Autodesk Inventor part; units mm, degrees
ref_plane "YZ Plane" through (0, 0, 0) normal (1, 0, 0) x (0, 1, 0)
ref_plane "XZ Plane" through (0, 0, 0) normal (0, 1, 0) x (-1, 0, 0)
ref_plane "XY Plane" through (0, 0, 0) normal (0, 0, 1) x (1, 0, 0)
sketch "Sketch1" plane through (0, 0, 0) normal (0, 0, 1) x (1, 0, 0)
  line L0 (0, 0) -> (25.4, 0)
  line L1 (25.4, 0) -> (25.4, 50.8)
  line L2 (25.4, 50.8) -> (0, 50.8)
  line L3 (0, 50.8) -> (0, 0)
  line L4 (22.86, 48.26) -> (22.86, 2.54)
  line L5 (22.86, 2.54) -> (2.54, 2.54)
  line L6 (2.54, 2.54) -> (2.54, 48.26)
  line L7 (2.54, 48.26) -> (22.86, 48.26)
  dimension "d0" = 25.4
  dimension "d1" = 50.8
  dimension "d2" = 2.54
extrude "Extrusion1" add sketch "Sketch1" along normal blind 711.2
sketch "Sketch2" plane through (0, 50.8, 0) normal (0, 1, 0) x (1, 0, 0)
  circle A0 centre (12.7, -12.7) radius 1.9844
  line L0 (25.4, 0) -> (0, 0)
  line L1 (25.4, 0) -> (25.4, -711.2)
  circle A1 centre (12.7, -38.1) radius 1.9844
  circle A2 centre (12.7, -63.5) radius 1.9844
  circle A3 centre (12.7, -88.9) radius 1.9844
  circle A4 centre (12.7, -114.3) radius 1.9844
  circle A5 centre (12.7, -139.7) radius 1.9844
  circle A6 centre (12.7, -165.1) radius 1.9844
  circle A7 centre (12.7, -190.5) radius 1.9844
  circle A8 centre (12.7, -215.9) radius 1.9844
  circle A9 centre (12.7, -241.3) radius 1.9844
  circle A10 centre (12.7, -266.7) radius 1.9844
  circle A11 centre (12.7, -292.1) radius 1.9844
  circle A12 centre (12.7, -317.5) radius 1.9844
  circle A13 centre (12.7, -342.9) radius 1.9844
  circle A14 centre (12.7, -368.3) radius 1.9844
  circle A15 centre (12.7, -393.7) radius 1.9844
  circle A16 centre (12.7, -419.1) radius 1.9844
  circle A17 centre (12.7, -444.5) radius 1.9844
  circle A18 centre (12.7, -469.9) radius 1.9844
  circle A19 centre (12.7, -495.3) radius 1.9844
  circle A20 centre (12.7, -520.7) radius 1.9844
  circle A21 centre (12.7, -546.1) radius 1.9844
  circle A22 centre (12.7, -571.5) radius 1.9844
  circle A23 centre (12.7, -596.9) radius 1.9844
  circle A24 centre (12.7, -622.3) radius 1.9844
  circle A25 centre (12.7, -647.7) radius 1.9844
  circle A26 centre (12.7, -673.1) radius 1.9844
  circle A27 centre (12.7, -698.5) radius 1.9844
  circle A28 centre (12.7, -723.9) radius 1.9844
  dimension "d5" = 3.9688
  dimension "d6" = 12.7
  dimension "d7" = 12.7
  dimension "d10" = 25.4
extrude "Extrusion2" cut sketch "Sketch2" against normal blind 76.2
properties part number "28in OChannel 1x2" material "Aluminum 6061-AHC"
Here's how the part is built. I have some questions about the finished solid (model axes, mm). A direction names the side the tool comes from. Coordinates: 2 decimals unless noted, no trailing zeros. Order: outer loops, then holes, each group sorted by start corner. A loop starts at its lowest first (then second) coordinate and runs counter-clockwise, first axis right, second up.
1) We'd pull the mould along Y, two halves only. Please class faces 1 (the face through (13, 0, 351)), 2 (the face through (13, 2.54, 351)), 3 (the face through (25.4, 25, 351)), 4 (the face through (13, 48.26, 351)): +Y half, -Y half, draft (parallel to the pull), parting line (faces both ways), or undercut.
2) I need wall thicknesses on line 1 (Y direction, x = 10, z = 497); line 2 (X direction, y = 49.9, z = 88.9); line 3 (X direction, y = 41.5, z = 168.5). Which ranges of each line are inside material? Lowest first, please.
3) Which directions (+Z, -Z, +X, -X, +Y, -Y) give clear straight access to the entire face, cutting with the end or side of a thin tool? Please do faces 5 (the face through (22.86, 26, 351)), 6 (the face through (13, 50.8, 351)).
4) Imagine slicing it at A-A on y = 41.5. List the corners of the cut face in (x, z) for me, and give its area (3 significant figures).
Response values:
1. face 1: -Y half
1. face 2: undercut
1. face 3: draft
1. face 4: undercut
2. line 1: y = 0 to 2.54, 48.26 to 50.8
2. line 2: x = 0 to 10.72, 14.68 to 25.4
2. line 3: x = 0 to 2.54, 22.86 to 25.4
3. face 5: +Z, -Z
3. face 6: +Z, -Z, +X, -X, +Y
4. outline: (0, 0) - (2.54, 0) - (2.54, 711.2) - (0, 711.2) - close; (22.86, 0) - (25.4, 0) - (25.4, 711.2) - (22.86, 711.2) - close
4. area: 3,610 mm2
